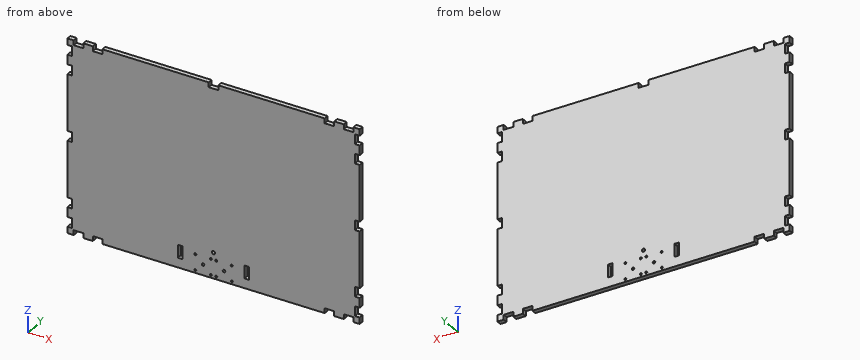
```python
from build123d import *

# Parameters (mm, degrees)
SKETCH1_W           = 584.2
SKETCH1_H           = 381
BOSS_EXTRUDE1_DEPTH = 9.525
SKETCH2_W           = 9.525
SKETCH2_H           = 19.05
SKETCH2_W_2         = 19.05
SKETCH2_H_2         = 9.525
CUT_EXTRUDE1_DEPTH  = 698.525172037
SKETCH3_R           = 2.032
SKETCH3_R_2         = 2.54
SKETCH3_R_3         = 3.175
SKETCH3_W           = 9.525
SKETCH3_H           = 25.4
CUT_EXTRUDE2_DEPTH  = 698.525172037


with BuildPart() as part:
    # Sketch1 → Boss-Extrude1 (new body)
    with BuildSketch(Plane(origin=(0, 0, 0), x_dir=(1, 0, 0), z_dir=(0, 1, 0))):
        with Locations((292.1, 190.5)):
            Rectangle(SKETCH1_W, SKETCH1_H)
    extrude(amount=BOSS_EXTRUDE1_DEPTH)

    # Sketch2 → Cut-Extrude1 (cut, through all)
    with BuildSketch(Plane(origin=(0, 9.525, 0), x_dir=(1, 0, 0), z_dir=(0, 1, 0))):
        with Locations((4.7625, 358.775)):
            Rectangle(SKETCH2_W, SKETCH2_H)
        with Locations((22.225, 376.2375)):
            Rectangle(SKETCH2_W_2, SKETCH2_H_2)
        with Locations((561.975, 376.2375)):
            Rectangle(SKETCH2_W_2, SKETCH2_H_2)
        with Locations((579.4375, 358.775)):
            Rectangle(SKETCH2_W, SKETCH2_H)
        with Locations((579.4375, 22.225)):
            Rectangle(SKETCH2_W, SKETCH2_H)
        with Locations((561.975, 4.7625)):
            Rectangle(SKETCH2_W_2, SKETCH2_H_2)
        with Locations((4.7625, 22.225)):
            Rectangle(SKETCH2_W, SKETCH2_H)
        with Locations((22.225, 4.7625)):
            Rectangle(SKETCH2_W_2, SKETCH2_H_2)
        with Locations((292.1, 4.7625)):
            Rectangle(SKETCH2_W_2, SKETCH2_H_2)
        with Locations((4.7625, 190.5)):
            Rectangle(SKETCH2_W, SKETCH2_H)
        with Locations((579.4375, 190.5)):
            Rectangle(SKETCH2_W, SKETCH2_H)
        with Locations((60.325, 376.2375)):
            Rectangle(SKETCH2_W_2, SKETCH2_H_2)
        with Locations((4.7625, 320.675)):
            Rectangle(SKETCH2_W, SKETCH2_H)
        with Locations((523.875, 376.2375)):
            Rectangle(SKETCH2_W_2, SKETCH2_H_2)
        with Locations((579.4375, 320.675)):
            Rectangle(SKETCH2_W, SKETCH2_H)
        with Locations((579.4375, 60.325)):
            Rectangle(SKETCH2_W, SKETCH2_H)
        with Locations((523.875, 4.7625)):
            Rectangle(SKETCH2_W_2, SKETCH2_H_2)
        with Locations((4.7625, 60.325)):
            Rectangle(SKETCH2_W, SKETCH2_H)
        with Locations((60.325, 4.7625)):
            Rectangle(SKETCH2_W_2, SKETCH2_H_2)
    extrude(amount=-CUT_EXTRUDE1_DEPTH, mode=Mode.SUBTRACT)

    # Sketch3 → Cut-Extrude2 (cut, through all)
    with BuildSketch(Plane(origin=(0, 9.525, 0), x_dir=(1, 0, 0), z_dir=(0, 1, 0))):
        with Locations(Location((255.651, 375.412, 0), (0, 0, 270))):
            Circle(SKETCH3_R)
        with Locations(Location((328.549, 375.412, 0), (0, 0, 270))):
            Circle(SKETCH3_R)
        with Locations(Location((286.639, 375.412, 0), (0, 0, 270))):
            Circle(SKETCH3_R)
        with Locations(Location((297.561, 375.412, 0), (0, 0, 270))):
            Circle(SKETCH3_R)
        with Locations(Location((255.651, 344.424, 0), (0, 0, 270))):
            Circle(SKETCH3_R)
        with Locations(Location((286.639, 344.424, 0), (0, 0, 270))):
            Circle(SKETCH3_R)
        with Locations(Location((297.561, 344.424, 0), (0, 0, 270))):
            Circle(SKETCH3_R)
        with Locations(Location((328.549, 344.424, 0), (0, 0, 270))):
            Circle(SKETCH3_R)
        with Locations(Location((271.145, 359.918, 0), (0, 0, 270))):
            Circle(SKETCH3_R_2)
        with Locations(Location((313.055, 359.918, 0), (0, 0, 270))):
            Circle(SKETCH3_R_2)
        with Locations(Location((292.1, 330.2, 0), (0, 0, 270))):
            Circle(SKETCH3_R_3)
        with Locations((358.7115, 349.25)):
            Rectangle(SKETCH3_W, SKETCH3_H)
        with Locations((225.4885, 349.25)):
            Rectangle(SKETCH3_W, SKETCH3_H)
    extrude(amount=-CUT_EXTRUDE2_DEPTH, mode=Mode.SUBTRACT)


solid = part.part
```
Geometry: final body of the model. Coordinates: model frame, mm. Coordinates: 2 decimals unless noted, no trailing zeros.
Item 1: Contact query for a flat-ended pin moving along its axis: P1, Ø5, axis at y = 5, z = -23.5, coming from the -X side (3 decimals). Output: stop coordinate, or through.
Answer:
P1: stops at x = 9.525
Item 2: Section query A-A (y = 4). State how many separate pieces and enclosed holes the cut face has, then the cut area to 3 significant figures.
Answer:
separate pieces: 1
enclosed holes: 13
area: 218,000 mm2
Item 3: Material intervals for line 1 along Z through (x, y) = (526, 3) (3 decimals); line 2 along X through (y, z) = (8.25, -60) (3 decimals), sorted ascending.
Answer:
line 1: z = -371.475 to -9.525
line 2: x = 9.525 to 574.675
